from build123d import *

# Parameters (mm, degrees)
F0_W     = 170
F0_H     = 170
F1_DEPTH = 100
F2_R     = 7.5
F3_DEPTH = 25
F4_R     = 5
F5_R     = 5
F6_W     = 50
F6_H     = 30
F6_W_2   = 30
F6_H_2   = 50
F7_DEPTH = 5


with BuildPart() as f1:
    # F0 (on Top) → F1 (new body)
    with BuildSketch(Plane.XY):
        Rectangle(F0_W, F0_H)
    extrude(amount=F1_DEPTH)

    # F2 (on face) → F3 (cut)
    with BuildSketch(Plane(origin=(0, 0, 0), x_dir=(1, 0, 0), z_dir=(0, 0, -1))):
        Circle(F2_R)
        Polygon((-60, 77.320508), (-75, 68.660254), (-75, 51.339746), (-60, 42.679492), (-45, 51.339746), (-45, 68.660254), align=None)
        Polygon((60, -77.320508), (75, -68.660254), (75, -51.339746), (60, -42.679492), (45, -51.339746), (45, -68.660254), align=None)
    extrude(amount=-F3_DEPTH, mode=Mode.SUBTRACT)

    # F4
    f4_edges = [f1.edges().sort_by_distance(p)[0] for p in [
        (-85, -85, 50),
        (85, -85, 50),
        (85, 85, 50),
        (-85, 85, 50),
    ]]
    fillet(f4_edges, radius=F4_R)

    # F5
    f5_edges = [f1.edges().sort_by_distance(p)[0] for p in [
        (0, -85, 100),
        (85, 0, 0),
    ]]
    fillet(f5_edges, radius=F5_R)

    # F6 (on face) → F7 (join)
    with BuildSketch(Plane(origin=(0, 0, 0), x_dir=(1, 0, 0), z_dir=(0, 0, -1))):
        with Locations((0, 42)):
            Rectangle(F6_W, F6_H)
        with Locations((42, 0)):
            Rectangle(F6_W_2, F6_H_2)
        with Locations((-42, 0)):
            Rectangle(F6_W_2, F6_H_2)
        with Locations((0, -42)):
            Rectangle(F6_W, F6_H)
    extrude(amount=F7_DEPTH)


solid = f1.part
Build history of the part. All positions in model axes, mm. A direction names the side the tool comes from. Coordinates: 2 decimals unless noted, no trailing zeros. Order: outer loops, then holes, each group sorted by start corner. A loop starts at its lowest first (then second) coordinate and runs counter-clockwise, first axis right, second up. Notation, with made-up numbers: M 34.5,84 L 73.5,84 A11 ccw 73.5,98 Z; hole C -32,48 d1. An arc over 180 degrees is marked long. One line per question, with ' | ' between items. Start each with the question number.
Q1. 3-axis set-ups, long thin cutter, end or side, ignore diameter. For faces 5 (the face through (-52.6, -46.95, 12.32)), 6 (the face through (0, -57, -2)), 7 (the face through (-25, 42, -2)), 8 (the face through (-42, 0, -5)), 9 (the face through (0, 57, -2)): which of +Z, -Z, +X, -X, +Y, -Y reach the whole face in a straight line?
Q2. Saw through at A-A (z = 18). List the corners of the cut face in (x, y).
Q3. Flat gauge pins, fed straight in: pin 1 Ø4 at (y, z) = (38.5, -1.5) entering from +X; pin 2 Ø5.5 at (x, z) = (-48.5, -1.5) entering from +Y; pin 3 Ø24 at (x, y) = (58, 53) entering from -Z. Where does each tip first touch, or does it go through?
Q4. Saw through at B-B (x = 0). List the corners of the cut face in (y, z), then the cut area to 3 significant figures.
Q5. Two-plate mould, pull along X, no slides. Class faces 1 (the face through (-27, 0, -2)), 2 (the face through (83, 1, 99)), 3 (the face through (-1, 83, 1)), 4 (the face through (45, 60, 12)): +X half, -X half, draft (parallel to the pull), parting line (faces both ways), or undercut.
Q6. Saw through at C-C (y = 32.5). List the corners of the cut face in (x, z).
Q7. Probe L1, parallel to Y at x = 0, z = 9.25; L2, parallel to Z at x = 46, y = -77; L3, parallel to Y at x = -60, z = 22. List the from-to ranges inside material, lowest first. Write a range as from..to.
Check values:
1) face 5: -Z | face 6: -Z, +X, -X, -Y | face 7: -Z, -X, +Y, -Y | face 8: -Z, +X, -X, +Y, -Y | face 9: -Z, +X, -X, +Y
2) outline: M -85,-80 A5 ccw -80,-85 L 80,-85 A5 ccw 85,-80 L 85,80 A5 ccw 80,85 L -80,85 A5 ccw -85,80 Z; hole M -75,-68.66 L -60,-77.32 L -45,-68.66 L -45,-51.34 L -60,-42.68 L -75,-51.34 Z; hole C 0,0 d15; hole M 45,51.34 L 60,42.68 L 75,51.34 L 75,68.66 L 60,77.32 L 45,68.66 Z
3) pin 1: stops at x = 82.18 | pin 2: stops at y = 83.31 | pin 3: stops at z = 0
4) outline: M -85,5 A5 ccw -80,0 L -57,0 L -57,-5 L -27,-5 L -27,0 L -7.5,0 L -7.5,25 L 7.5,25 L 7.5,0 L 27,0 L 27,-5 L 57,-5 L 57,0 L 80,0 A5 ccw 85,5 L 85,95 A5 ccw 80,100 L -80,100 A5 ccw -85,95 Z | area: 16,900 mm2
5) face 1: undercut | face 2: +X half | face 3: draft | face 4: undercut
6) outline: M -85,5 A5 ccw -80,0 L -25,0 L -25,-5 L 25,-5 L 25,0 L 80,0 A5 ccw 85,5 L 85,95 A5 ccw 80,100 L -80,100 A5 ccw -85,95 Z
7) L1: y = -85..-7.5, 7.5..85 | L2: z = 0..100 | L3: y = -85..-77.32, -42.68..85
